Study the drawing (mm; zero at the part's minimum x, y, z) and answer. A direction names the side the tool comes from. Round coordinates to 2 decimals unless told otherwise and drop trailing zeros. Write each loop counter-clockwise with the first axis right and the second up, starting at its lowest first coordinate (ties: lowest second). Pieces come first, ordered by that corner, then holes. Notation, with made-up numbers: M 19.5,30 L 74.5,30 A29 cw 74.5,56 Z; hole C -39.75,42.5 d6. An arc over 180 degrees is marked long. Put each result on its own line as item: value. Start each with the question number.
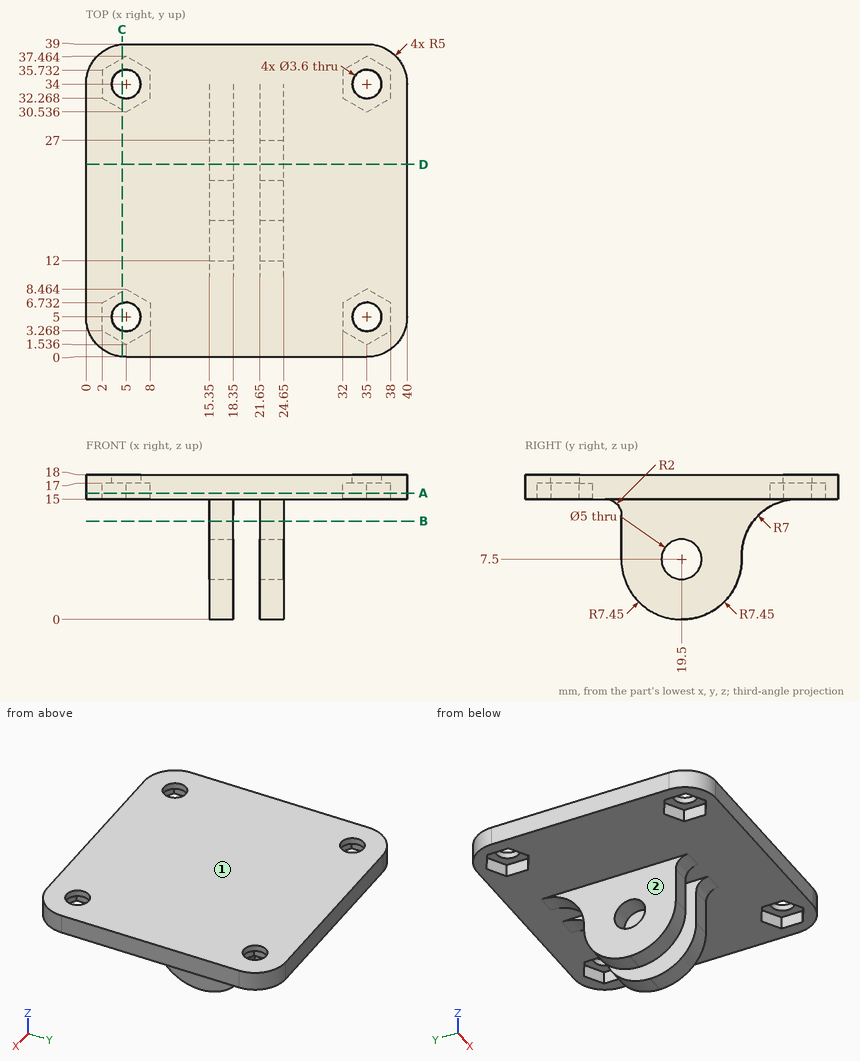
Item 1: Section C-C (x = 4.5) is taken. Give the vertices of the cut face in (y, z) (1 decimal).
Item 2: Section D-D (y = 24) is taken. Give the vertices of the cut face in (x, z) (3 decimals).
Item 3: Flat-ended cylindrical pins translate along their axes: pin 1 (11.5 mm diameter, centred on x = 15.5, y = 22.5, fed in from -Z); pin 2 (6.5 mm diameter, centred on x = 4, y = 6.5, fed in from -Z); pin 3 (0.6 mm diameter, centred on y = 4.5, z = 16, fed in from -X); pin 4 (6.5 mm diameter, centred on y = 19.5, z = 7.5, fed in from +X). Find the tip coordinate at first contact, or state that the pin passes through.
Item 4: Which of the six approach directions +Z, -Z, +X, -X, +Y, -Y give full straight-line access (tool end or side, diameter ignored) to the marked faces 1 and 2?
Item 5: Section A-A (z = 15.75) is taken. Count the separate pieces of the cut face and the enclosed holes in it, and give its area (3 significant figures).
Item 6: Section B-B (z = 12.25) is taken. Give the vertices of the cut face in (x, y).
Item 7: Consider line 1 along Y through (x, z) = (22.3, 7.5); line 2 along X through (y, z) = (15.5, 11.5); line 3 along Z through (x, y) = (12, 11.5). Determine where each line is inside the solid, lowest interval first. Write a range as [from, to].
Output values:
1. outline: M 0,15 L 1.8,15 L 1.8,17 L 3.3,17 L 3.3,18 L 0,18 Z; M 6.7,17 L 8.2,17 L 8.2,15 L 30.8,15 L 30.8,17 L 32.3,17 L 32.3,18 L 6.7,18 Z; M 35.7,17 L 37.2,17 L 37.2,15 L 39,15 L 39,18 L 35.7,18 Z
2. outline: M 0,15 L 15.35,15 L 15.35,1.475 L 18.35,1.475 L 18.35,15 L 21.65,15 L 21.65,1.475 L 24.65,1.475 L 24.65,15 L 40,15 L 40,18 L 0,18 Z
3. pin 1: stops at z = 0
3. pin 2: stops at z = 15
3. pin 3: stops at x = 0
3. pin 4: stops at x = 24.65
4. face 1: +Z, +X, -X, +Y, -Y
4. face 2: -Z, -X, +Y, -Y
5. separate pieces: 1
5. enclosed holes: 4
5. area: 1,410 mm^2
6. outline: M 15.35,12 L 18.35,12 L 18.35,28.44 L 15.35,28.44 Z; M 21.65,12 L 24.65,12 L 24.65,28.44 L 21.65,28.44 Z
7. line 1: y = [12, 17], [22, 27]
7. line 2: x = [15.35, 18.35], [21.65, 24.65]
7. line 3: z = [15, 18]
